from build123d import *

# Parameters (mm, degrees)
F0_W     = 8
F0_H     = 8
F0_R     = 2
F1_DEPTH = 1
F0_R_2   = 5
F2_DEPTH = 6.6
F3_R     = 5
F3_R_2   = 3.272318
F4_DEPTH = 1
F5_SIZE  = 1


with BuildPart() as f1:
    # F0 (on Top) → F1 (new body)
    with BuildSketch(Plane.XY):
        with Locations((-9, 11.880489)):
            Rectangle(F0_W, F0_H)
        with Locations((-9, 11.880489)):
            Circle(F0_R, mode=Mode.SUBTRACT)
        with BuildLine():
            ThreePointArc((-6.154522, -2.467193), (-6.302399, 2.06033), (-3.508691, 5.626214))
            Line((-3.508691, 5.626214), (-5, 7.880489))
            Line((-5, 7.880489), (-13, 7.880489))
            Line((-13, 7.880489), (-6.154522, -2.467193))
        make_face()
    extrude(amount=F1_DEPTH)

    # F0 (on Top) → F2 (join)
    with BuildSketch(Plane.XY):
        with BuildLine():
            ThreePointArc((-6.154522, -2.467193), (1.256356, -6.510512), (6.630625, 0))
            ThreePointArc((6.630625, 0), (3.217171, 5.797845), (-3.508691, 5.626214))
            ThreePointArc((-3.508691, 5.626214), (-6.302399, 2.06033), (-6.154522, -2.467193))
        make_face()
        Circle(F0_R_2, mode=Mode.SUBTRACT)
    extrude(amount=F2_DEPTH)

    # F3 (on face) → F4 (join)
    with BuildSketch(Plane.XY.offset(6.6)):
        Circle(F3_R)
        Circle(F3_R_2, mode=Mode.SUBTRACT)
    extrude(amount=-F4_DEPTH)

    # F5
    f5_edges = [f1.edges().sort_by_distance(p)[0] for p in [
        (3.508691, -5.626214, 6.6),
    ]]
    chamfer(f5_edges, length=F5_SIZE)


solid = f1.part
Part model, mm, in its own coordinate system. A direction names the side the tool comes from. Round coordinates to 2 decimals unless told otherwise and drop trailing zeros. Write each loop counter-clockwise with the first axis right and the second up, starting at its lowest first coordinate (ties: lowest second). Pieces come first, ordered by that corner, then holes. Notation, with made-up numbers: (7, 69.5) - (34, 69.5) arc R16 ccw to (34, 83.5) - close; hole circle Ø7 at (60, 32). An arc over 180 degrees is marked (long way). Use CSV: the item, a comma, the result in double quotes.
Item 1: Slice it at A-A, the plane x = -9. Write the cut outline in (y, z).
Results list:
outline,"(1.83, 0) - (9.88, 0) - (9.88, 1) - (1.83, 1) - close; (13.88, 0) - (15.88, 0) - (15.88, 1) - (13.88, 1) - close"
Item 2: Flat gauge pins, fed straight in: P1, Ø1, axis at y = 4, z = 1, coming from the -X side; P2, Ø3, axis at x = -4.5, y = 7.5, coming from the +Z side; P3, Ø1.1, axis at y = 13.5, z = 0.5, coming from the +X side. Where does each tip first touch, or does it go through?
Results list:
P1,"stops at x = -10.76"
P2,"stops at z = 1"
P3,"stops at x = -5"
Item 3: Tool access for faces 1 (the flat face through (-4.244, 6.738, 0.493)), 2 (the flat face through (3.3, -1, 5.6)), 3 (the flat face through (-13, 11.8, 0.5)), 4 (the flat face through (-5, 11.8, 0.5)): list every direction of +Z, -Z, +X, -X, +Y, -Y with a clear straight run to the whole face (end or side of a thin tool).
Results list:
face 1,"+Z, -Z, +Y"
face 2,"-Z"
face 3,"+Z, -Z, -X, +Y, -Y"
face 4,"+Z, -Z, +X, +Y"
Item 4: Wall check: L1, parallel to Y at x = 0, z = 4.25; L2, parallel to Z at x = -4.5, y = 0.75; L3, parallel to Z at x = -7, y = 13.25. Give the ranges that are in metal, low to high.
Results list:
L1,"y = -6.63 to -5, 5 to 6.63"
L2,"z = 5.6 to 6.6"
L3,"z = 0 to 1"
Item 5: Pull direction X, two halves, no side cores. Call faces 5 (the flat face through (-9.625, 2.779, 0.493)), 6 (the flat face through (-6, 5, 0)), 7 (the cylindrical face through (-9.26, 13.863, 0.493)), 8 (the cylindrical face through (-1.08, -4.88, 2.76)): pulls with the +X half, pulls with the -X half, needs draft (parallel to the pull), parting line crosses it, or undercut.
Results list:
face 5,"pulls with the -X half"
face 6,"needs draft"
face 7,"undercut"
face 8,"undercut"
Item 6: Slice it at B-B, the plane z = 4.25. Write the cut outline in (x, y), then the cut area to 3 significant figures.
Results list:
outline,"(-6.15, -2.47) arc R6.63 ccw to (6.63, 0) arc R6.63 ccw (long way) to start; hole circle Ø10 at (0, 0)"
area,"59.6 mm²"
Item 7: Slice it at C-C, the plane x = -11.5. Write the cut outline in (y, z).
Results list:
outline,"(5.61, 0) - (15.88, 0) - (15.88, 1) - (5.61, 1) - close"
